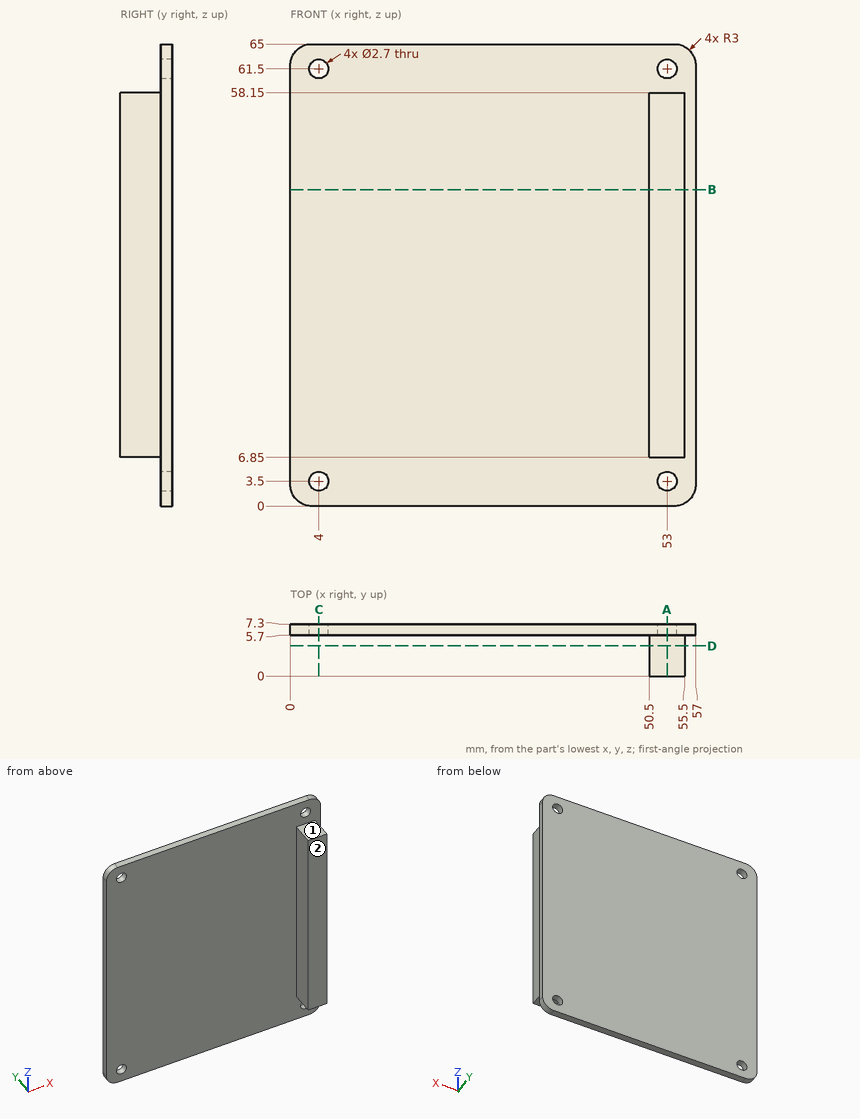
Study the drawing (mm; zero at the part's minimum x, y, z) and answer. A direction names the side the tool comes from. Coordinates: 2 decimals unless noted, no trailing zeros. Loops run counter-clockwise (first coordinate to the right, second up) from the corner with the lowest first, then second, coordinate; pieces in that order, holes last. Notation, with made-up numbers: M -9.75,34.25 L 47.25,34.25 A29 cw 47.25,72.25 Z; hole C -8,20 d9. An arc over 180 degrees is marked long. Answer in a Markdown table with one row per item.
1) Find the intervals of material crossed by probe 1 along X at (y, z) = (6.4, 3.5); probe 2 along Y at (x, z) = (11, 23); probe 3 along X at (y, z) = (2.75, 39.5), in increasing order.
Answers below:
| item | result |
|---|---|
| probe 1 | 0 to 2.65, 5.35 to 51.65, 54.35 to 57 |
| probe 2 | 5.7 to 7.3 |
| probe 3 | 50.5 to 55.5 |
2) Given pin 1 (1.5 mm diameter, centred on x = 54, y = 3, fed in from +Z); pin 2 (3.5 mm diameter, centred on x = 53, z = 3.5, fed in from -Y); pin 3 (2 mm diameter, centred on x = 53, z = 61.5, fed in from -Y); pin 4 (1.7 mm diameter, centred on y = 3, z = 40.5, fed in from -X), each flat-ended and moving along its own axis, determine where each tip first touches the part or whether it passes through.
Answers below:
| item | result |
|---|---|
| pin 1 | z = 58.15 |
| pin 2 | y = 5.7 |
| pin 3 | through |
| pin 4 | x = 50.5 |
3) Find section B-B (z = 44.5). Determine the outline of the cut face in (x, y).
Answers below:
| item | result |
|---|---|
| outline | M 0,5.7 L 50.5,5.7 L 50.5,0 L 55.5,0 L 55.5,5.7 L 57,5.7 L 57,7.3 L 0,7.3 Z |
4) Find section A-A (x = 53). Determine the outline of the cut face in (y, z), then the cut area to 3 significant figures.
Answers below:
| item | result |
|---|---|
| outline | M 0,6.85 L 5.7,6.85 L 5.7,4.85 L 7.3,4.85 L 7.3,60.15 L 5.7,60.15 L 5.7,58.15 L 0,58.15 Z; M 5.7,0 L 7.3,0 L 7.3,2.15 L 5.7,2.15 Z; M 5.7,62.85 L 7.3,62.85 L 7.3,65 L 5.7,65 Z |
| area | 388 mm^2 |
5) Find section C-C (x = 4). Determine the outline of the cut face in (y, z).
Answers below:
| item | result |
|---|---|
| outline | M 5.7,0 L 7.3,0 L 7.3,2.15 L 5.7,2.15 Z; M 5.7,4.85 L 7.3,4.85 L 7.3,60.15 L 5.7,60.15 Z; M 5.7,62.85 L 7.3,62.85 L 7.3,65 L 5.7,65 Z |
6) Find section D-D (y = 4.25). Determine the outline of the cut face in (x, z).
Answers below:
| item | result |
|---|---|
| outline | M 50.5,6.85 L 55.5,6.85 L 55.5,58.15 L 50.5,58.15 Z |
7) Which of the six approach directions +Z, -Z, +X, -X, +Y, -Y give full straight-line access (tool end or side, diameter ignored) to the marked faces 1 and 2?
Answers below:
| item | result |
|---|---|
| face 1 | +Z, +X, -X, -Y |
| face 2 | +Z, -Z, +X, -X, -Y |
